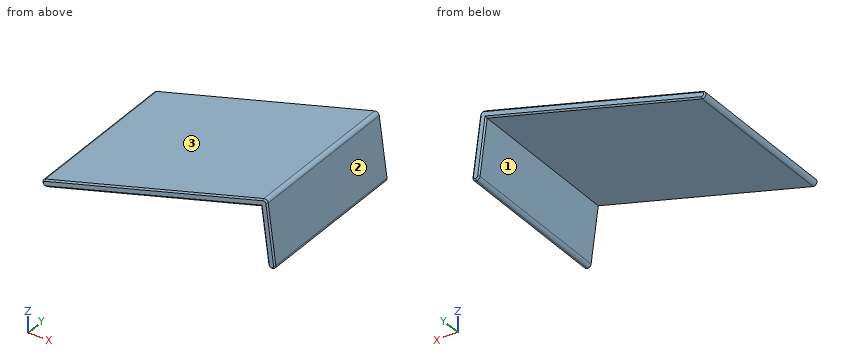
from build123d import *

# Parameters (mm, degrees)
F1_DEPTH = 118
F2_SIZE  = 1


with BuildPart() as f1:
    # F0 (on Front) → F1 (new body)
    with BuildSketch(Plane.XZ):
        with BuildLine():
            ThreePointArc((-12.9717128781, 4.9148145657), (-14.8032774188, 2.1736845194), (-12.3246652653, 0))
            Line((-12.3246652653, 0), (-11.9955340214, 0))
            Line((-11.9955340214, 0), (140.1169462795, 40.7584162553))
            Line((140.1169462795, 40.7584162553), (145.1967225812, 2.1736845194))
            ThreePointArc((145.1967225812, 2.1736845194), (146.0269701969, 0.6204004813), (147.6753347347, 0))
            ThreePointArc((147.6753347347, 0), (149.5549342534, 0.8516354622), (150.1539468881, 2.8263154806))
            Line((150.1539468881, 2.8263154805), (144.7020790944, 44.237362697))
            ThreePointArc((144.7020790944, 44.237362697), (143.6123925235, 45.9897212472), (141.5764193282, 46.3258617821))
            Line((141.5764193282, 46.3258617821), (-12.9717128781, 4.9148145657))
        make_face()
    extrude(amount=F1_DEPTH)

    # F2
    f2_edges = [f1.edges().sort_by_distance(p)[0] for p in [
        (64.302353, -118, 25.620338),
        (-14.803277, -118, 2.173685),
        (-12.1601, -118, 0),
        (64.060706, -118, 20.379208),
        (142.656834, -118, 21.46605),
        (148.00165, -118, 0.021388),
        (147.428013, -118, 23.531839),
        (143.612393, -118, 45.989721),
        (64.302353, 0, 25.620338),
        (-14.803277, 0, 2.173685),
        (-12.1601, 0, 0),
        (64.060706, 0, 20.379208),
        (142.656834, 0, 21.46605),
        (148.00165, 0, 0.021388),
        (147.428013, 0, 23.531839),
        (143.612393, 0, 45.989721),
    ]]
    chamfer(f2_edges, length=F2_SIZE)


solid = f1.part
Could you check a few things on this model? Use its own coordinates, in mm. Face numbers are marked on the shaded views. Coordinates: 2 decimals unless noted, no trailing zeros. Write each loop counter-clockwise with the first axis right and the second up, starting at its lowest first coordinate (ties: lowest second). Pieces come first, ordered by that corner, then holes. Notation, with made-up numbers: M 42.5,66 L 62.5,66 A29 ccw 62.5,100 Z; hole C 4.5,78.25 d11. An arc over 180 degrees is marked long. One line per question, with ' | ' between items.
1) If we mould it in two halves opening along X, with no side actions, what happens to the marked faces 1, 2 and 3? For each: released by +X, released by -X, zero draft, split by the parting line, or undercut.
Checks:
face 1: undercut | face 2: released by +X | face 3: released by -X
2) Imagine slicing it at B-B, the plane y = -29.5. Write out the boundary of the cut face in (x, z), and give its area (3 significant figures).
Checks:
outline: M -12.97,4.91 A2.5 ccw -12.32,0 L -12,0 L 140.12,40.76 L 145.2,2.17 A2.5 ccw 150.15,2.83 L 144.7,44.24 A2.5 ccw 141.58,46.33 Z | area: 1,030 mm²
3) Imagine slicing it at A-A, the plane z = 22. Write out the boundary of the cut face in (x, y), and give its area (3 significant figures).
Checks:
outline: M 50.79,-117 L 54.65,-118 L 66.25,-118 L 70.11,-117 L 70.11,-1 L 66.25,0 L 54.65,0 L 50.79,-1 Z; M 142.59,-117 L 143.6,-118 L 146.62,-118 L 147.63,-117 L 147.63,-1 L 146.62,0 L 143.6,0 L 142.59,-1 Z | area: 2,860 mm²
4) For pin 1 Ø12 at (y, z) = (-38.5, 39) entering from +X; pin 2 Ø1 at (x, y) = (8, -88.5) entering from -Z; pin 3 Ø10 at (x, y) = (64.5, -44) entering from +Z; pin 4 Ø10 at (x, z) = (65.5, 11.5) entering from -Y, each with a flat end and sliding along its axis, tell me the tip position at first contact or that it passes through.
Checks:
pin 1: x = 146.18 | pin 2: z = 5.22 | pin 3: z = 27.01 | pin 4: through
5) Imagine slicing it at C-C, the plane x = 113. Write out the boundary of the cut face in (y, z), and give its area (3 significant figures).
Checks:
outline: M -118,34.53 L -117,33.49 L -1,33.49 L 0,34.53 L 0,37.63 L -1,38.67 L -117,38.67 L -118,37.63 Z | area: 609 mm²
6) I need wall thicknesses on probe 1 along Z at (x, y) = (-6.5, -110.5); probe 2 along Z at (x, y) = (120, -13). Which ranges of each line are inside material? Lowest first, please. Write a range as [from, to].
Checks:
probe 1: [1.47, 6.65] | probe 2: [35.37, 40.54]
